from build123d import *

# Parameters (mm, degrees)
EXTRUDE_1_DEPTH = 9
CHAMFER_1_SIZE  = 3
SKETCH_3_R      = 3
SKETCH_3_R_2    = 2.5
EXTRUDE_2_DEPTH = 1


with BuildPart() as part:
    # 草图1 → 凸台-拉伸1 (new body)
    with BuildSketch(Plane(origin=(0, 0, 0), x_dir=(1, 0, 0), z_dir=(0, 1, 0))):
        Polygon((-18.403562193, 20.210244745), (-25.474630004, 13.139176933), (-25.474630004, -14.918687443), (-18.403562193, -21.989755255), (9.654302184, -21.989755255), (16.725369996, -14.918687443), (16.725369996, 13.139176933), (9.654302184, 20.210244745), align=None)
    extrude(amount=EXTRUDE_1_DEPTH)

    # 倒角1
    chamfer_1_edges = [part.edges().sort_by_distance(p)[0] for p in [
        (-25.474630004, 9, 0.889755255),
        (-21.939096098, 9, 18.454221349),
        (-4.374630004, 9, 21.989755255),
        (13.18983609, 9, 18.454221349),
        (16.725369996, 9, 0.889755255),
        (13.18983609, 9, -16.674710839),
        (-4.374630004, 9, -20.210244745),
        (-21.939096098, 9, -16.674710839),
    ]]
    chamfer(chamfer_1_edges, length=CHAMFER_1_SIZE)

    # 草图3 → 凸台-拉伸2 (add)
    # profile 1 of 4: a face of its own
    with BuildSketch(Plane.XZ):
        with Locations(Location((9.434831814, 14.699217073, 0), (0, 0, 90))):
            Circle(SKETCH_3_R)
        with Locations(Location((9.434831814, 14.699217073, 0), (0, 0, 270))):
            Circle(SKETCH_3_R_2, mode=Mode.SUBTRACT)
    # profile 2 of 4: a face of its own
    with BuildSketch(Plane.XZ):
        with Locations(Location((9.434831814, -12.919706563, 0), (0, 0, 90))):
            Circle(SKETCH_3_R)
        with Locations(Location((9.434831814, -12.919706563, 0), (0, 0, 270))):
            Circle(SKETCH_3_R_2, mode=Mode.SUBTRACT)
    # profile 3 of 4: a face of its own
    with BuildSketch(Plane.XZ):
        with Locations(Location((-18.184091822, -12.919706563, 0), (0, 0, 90))):
            Circle(SKETCH_3_R)
        with Locations(Location((-18.184091822, -12.919706563, 0), (0, 0, 270))):
            Circle(SKETCH_3_R_2, mode=Mode.SUBTRACT)
    # profile 4 of 4: a face of its own
    with BuildSketch(Plane.XZ):
        with Locations(Location((-18.184091822, 14.699217073, 0), (0, 0, 90))):
            Circle(SKETCH_3_R)
        with Locations(Location((-18.184091822, 14.699217073, 0), (0, 0, 270))):
            Circle(SKETCH_3_R_2, mode=Mode.SUBTRACT)
    extrude(amount=EXTRUDE_2_DEPTH)


solid = part.part
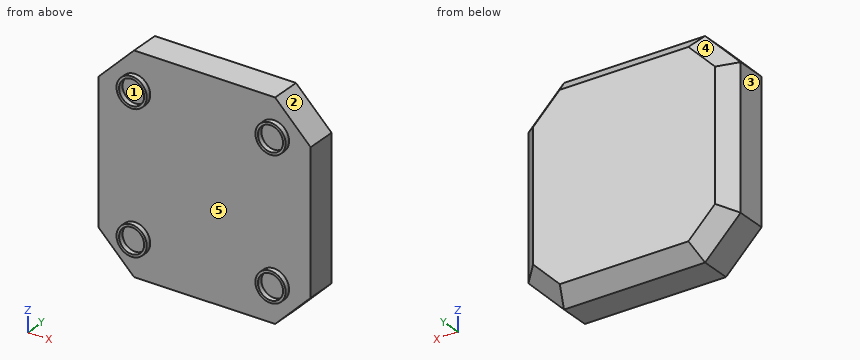
For this review, take the finished solid that the model builds, in its own axes (mm). Face numbers are marked on the shaded views. A direction names the side the tool comes from. Coordinates: 2 decimals unless noted, no trailing zeros. Order: outer loops, then holes, each group sorted by start corner. A loop starts at its lowest first (then second) coordinate and runs counter-clockwise, first axis right, second up. Notation, with made-up numbers: (-32.5, 18.5) -> (11.5, 18.5) arc R13 ccw to (11.5, 41.5) -> close; hole circle Ø3 at (19.25, -2). An arc over 180 degrees is marked (long way). Return JSON: item names as keys, results as strings.
1. We need section C-C on x = -14.5. Write out the cut boundary in (y, z).
Answer block:
{"outline": "(0, -20.21) -> (6, -20.21) -> (9, -17.21) -> (9, 18.99) -> (6, 21.99) -> (0, 21.99) -> close"}
2. We need section B-B on z = -6. Write out the cut boundary in (x, y), and give its area (3 significant figures).
Answer block:
{"outline": "(-25.47, 0) -> (16.73, 0) -> (16.73, 6) -> (13.73, 9) -> (-22.47, 9) -> (-25.47, 6) -> close", "area": "371 mm²"}
3. The part is to be moulded in two halves that separate along X. For the marked faces 1, 2 and 3, say which applies: +X half, -X half, draft (parallel to the pull), parting line (faces both ways), or undercut.
Answer block:
{"face 1": "undercut", "face 2": "+X half", "face 3": "-X half"}
4. Machinability: for the marked faces 4 and 5, which of the approach directions +Z, -Z, +X, -X, +Y, -Y give a long, thin tool a straight path to every point of the face, cutting with its end or side? Answer none if there is none.
Answer block:
{"face 4": "+Z, -X, +Y", "face 5": "-Y"}
5. For line 1 (Y direction, x = 11.5, z = 14); line 2 (Z direction, x = -12, y = 8.75); line 3 (X direction, y = 8, z = 5.5), list the stretches that pass through material, from the lowest coordinate up. Write a range as from..to.
Answer block:
{"line 1": "0..9", "line 2": "-17.46..19.24", "line 3": "-23.47..14.73"}
6. We need section D-D on y = 1.75. Write out the cut boundary in (x, z).
Answer block:
{"outline": "(-25.47, -13.14) -> (-18.4, -20.21) -> (9.65, -20.21) -> (16.73, -13.14) -> (16.73, 14.92) -> (9.65, 21.99) -> (-18.4, 21.99) -> (-25.47, 14.92) -> close"}
7. For pin 1 Ø2 at (x, z) = (-8, -12.5) entering from -Y, flat-tipped, find the tip position at first contact; note if it passes through.
Answer block:
{"pin 1": "y = 0"}
8. We need section A-A on y = -0.5. Write out the cut boundary in (x, z).
Answer block:
{"outline": "circle Ø6 at (-18.18, -12.92); circle Ø6 at (-18.18, 14.7); circle Ø6 at (9.43, -12.92); circle Ø6 at (9.43, 14.7); hole circle Ø5 at (-18.18, -12.92); hole circle Ø5 at (-18.18, 14.7); hole circle Ø5 at (9.43, -12.92); hole circle Ø5 at (9.43, 14.7)"}
